The model under review builds one solid part; all positions refer to its coordinate system, in mm. A direction names the side the tool comes from. Round coordinates to 2 decimals unless told otherwise and drop trailing zeros. Loops run counter-clockwise (first coordinate to the right, second up) from the corner with the lowest first, then second, coordinate; pieces in that order, holes last. Notation, with made-up numbers: M 11,0.5 L 39,0.5 A20 ccw 39,26.5 Z; hole C 10,37 d8. An arc over 180 degrees is marked long. One line per question, with ' | ' between items.
Autodesk Inventor part; units mm, degrees
ref_plane "YZ Plane" through (0, 0, 0) normal (1, 0, 0) x (0, 1, 0)
ref_plane "XZ Plane" through (0, 0, 0) normal (0, 1, 0) x (-1, 0, 0)
ref_plane "XY Plane" through (0, 0, 0) normal (0, 0, 1) x (1, 0, 0)
sketch "Sketch1" plane through (0, 0, 0) normal (0, 1, 0) x (-1, 0, 0)
  line L0 (50, 0) -> (44.5, 0)
  line L1 (44.5, 0) -> (44.5, 2)
  line L2 (44.5, 2) -> (34.5, 2)
  line L3 (34.5, 2) -> (34.5, 0)
  line L4 (34.5, 0) -> (15.5, 0)
  line L5 (15.5, 0) -> (15.5, 2)
  line L6 (15.5, 2) -> (5.5, 2)
  line L7 (5.5, 2) -> (5.5, 0)
  line L8 (5.5, 0) -> (0, 0)
  line L9 (0, 0) -> (0, -27.5)
  line L10 (0, -27.5) -> (50, -27.5)
  line L11 (50, -27.5) -> (50, 0)
  line L12 (50, -55) -> (44.5, -55)
  line L13 (44.5, -55) -> (44.5, -57)
  line L14 (44.5, -57) -> (34.5, -57)
  line L15 (34.5, -57) -> (34.5, -55)
  line L16 (34.5, -55) -> (15.5, -55)
  line L17 (15.5, -55) -> (15.5, -57)
  line L18 (15.5, -57) -> (5.5, -57)
  line L19 (5.5, -57) -> (5.5, -55)
  line L20 (5.5, -55) -> (0, -55)
  line L21 (0, -55) -> (0, -27.5)
  line L22 (50, -27.5) -> (50, -55)
  point P0 (0, -55)
  dimension "d1" = 50
  dimension "d2" = 10
  dimension "d3" = 10
  dimension "d4" = 5.5
  dimension "d5" = 5.5
  dimension "d6" = 2
  dimension "d7" = 27.5
extrude "Plate1" add sketch "Sketch1" along normal blind 2
equation "\"d8\" = Thickness"
equation "\"BendRadius\" = Thickness"
equation "\"BendReliefWidth\" = Thickness"
equation "\"BendReliefDepth\" = 0.5 * Thickness"
equation "\"CornerReliefSize\" = 4 * Thickness"
equation "\"MinimumRemnant\" = 2 * Thickness"
equation "\"TransitionRadius\" = BendRadius"
equation "\"JacobiRadiusSize\" = BendRadius"
equation "\"GapSize\" = Thickness"
properties part number "backstop_beslag"
1) Add section B-B on x = -28. State the section outline as (y, z) points, then the cut area to 3 significant figures.
Output values:
outline: M 0,-55 L 2,-55 L 2,0 L 0,0 Z | area: 110 mm²
2) Insertion check: P1, Ø1, axis at x = -21.5, y = 1.5, coming from the -Z side; P2, Ø1, axis at y = 0.5, z = -56, coming from the +X side; P3, Ø0.6, axis at x = -27, y = 1.5, coming from the +Z side. Each pin has a flat end and moves straight along its axis. Give the tip position at first contact, or say it passes through.
Output values:
P1: stops at z = -55 | P2: stops at x = -5.5 | P3: stops at z = 0
3) Mouldability with a two-part tool opening along X and no side actions: class faces 1 (the flat face through (0, 1, -27)), 2 (the flat face through (-34.5, 1, 1)), 3 (the flat face through (-25, 1, 0)), 4 (the flat face through (-25, 2, -27)) as +X half, -X half, draft (parallel to the pull), parting line (faces both ways), or undercut.
Output values:
face 1: +X half | face 2: undercut | face 3: undercut | face 4: draft
4) Add section A-A on y = 1.65. State the section outline as (x, z) points, then the cut area to 3 significant figures.
Output values:
outline: M -50,-55 L -44.5,-55 L -44.5,-57 L -34.5,-57 L -34.5,-55 L -15.5,-55 L -15.5,-57 L -5.5,-57 L -5.5,-55 L 0,-55 L 0,0 L -5.5,0 L -5.5,2 L -15.5,2 L -15.5,0 L -34.5,0 L -34.5,2 L -44.5,2 L -44.5,0 L -50,0 Z | area: 2,830 mm²
5) Machinability: for faces 5 (the flat face through (-5.5, 1, -56)), 6 (the flat face through (-44.5, 1, 1)), 7 (the flat face through (-5.5, 1, 1)), 8 (the flat face through (-47, 1, -55)), 9 (the flat face through (-15.5, 1, -56)), which of the approach directions +Z, -Z, +X, -X, +Y, -Y give a long, thin tool a straight path to every point of the face, cutting with its end or side? Answer none if there is none.
Output values:
face 5: -Z, +X, +Y, -Y | face 6: +Z, -X, +Y, -Y | face 7: +Z, +X, +Y, -Y | face 8: -Z, -X, +Y, -Y | face 9: -Z, +Y, -Y
6) For line 1 (Z direction, x = -4, y = 0.9), list the stretches that pass through material, from the lowest coordinate up.
Output values:
line 1: z = -55 to 0
